Design review of the part shown in the three views and the two pictorial views. Dimensions are in mm from the part's minimum x, y and z. A direction names the side the tool comes from. Give positions to 0.01 mm unless a question says otherwise; leave off trailing zeros. Loops run counter-clockwise (first coordinate to the right, second up) from the corner with the lowest first, then second, coordinate; pieces in that order, holes last. Notation, with made-up numbers: (46.25, 86) -> (99.25, 86) arc R10 cw to (99.25, 91) -> close; hole circle Ø2 at (-25, 40). An arc over 180 degrees is marked (long way). One line per question, with ' | ' between items. Start each with the question number.
(1) Consider section C-C (z = 17.25). Write out the cut boundary in (x, y), and give its area (3 significant figures).
(2) Consider section D-D (z = 12.25). Write out the cut boundary in (x, y) (3 decimals).
(3) Wall thickness on probe 1 along Z at (x, y) = (19.37, 0.85); probe 2 along X at (y, z) = (0.4, 7.25); probe 3 along Z at (x, y) = (14.37, 1.05) (3 decimals): over which ranges is each line inside the solid? List them lowest first.
(4) Consider section A-A (y = 5.75). Write out the cut boundary in (x, z), and give its area (3 significant figures).
(5) Insertion check: P1, Ø8, axis at x = 12, z = 36.5, coming from the +Y side; P2, Ø0.5, axis at x = 1, z = 26, coming from the +Y side. Each pin has a flat end and moves straight along its axis. Give the tip position at first contact, or say it passes through.
(6) Draft analysis for pull direction X (two halves, no side actions). For the marked faces 3, 4, 5 and 6, state which applies: +X half, -X half, draft (parallel to the pull), parting line (faces both ways), or undercut.
(7) Tool access review of the marked faces 1 and 2: name each direction out of +Z, -Z, +X, -X, +Y, -Y from which nothing blocks a thin tool from reaching the whole face with its end or side.
(8) Consider section B-B (x = 14.37). Write out the cut boundary in (y, z) (3 decimals).
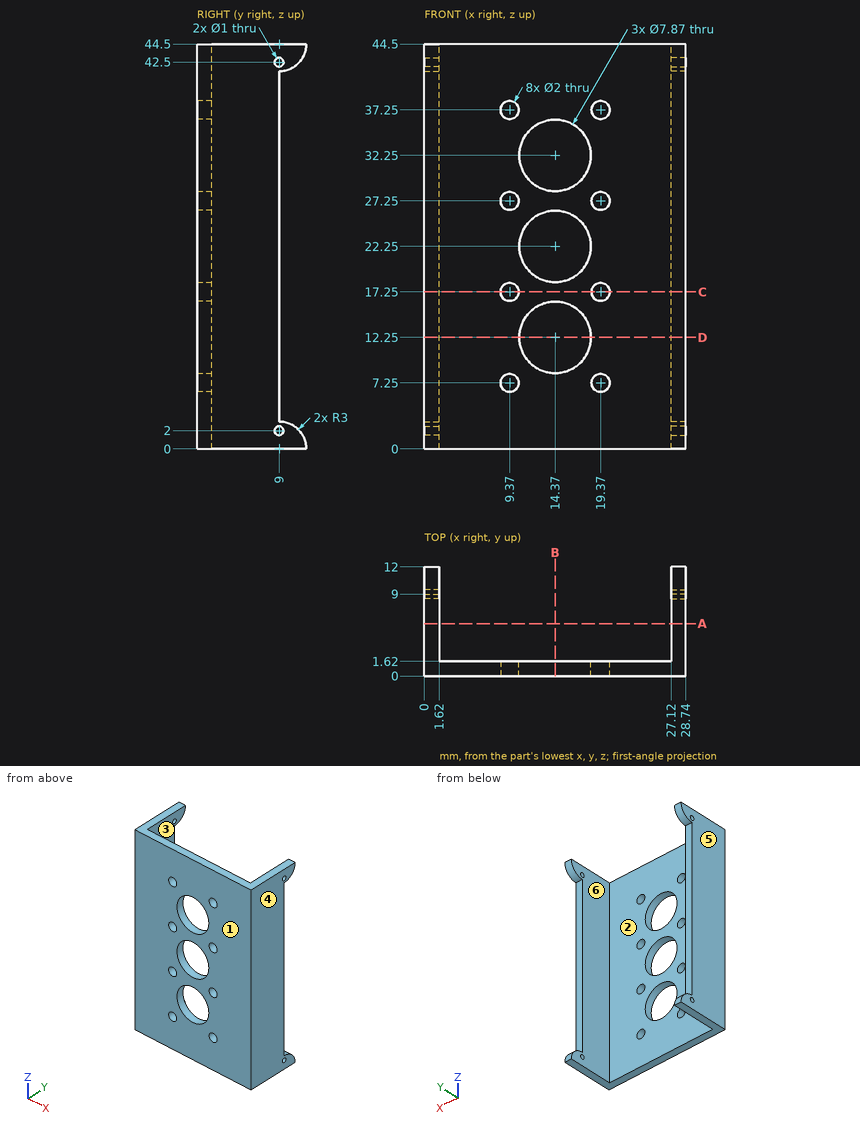
A:
1) outline: (0, 0) -> (8.37, 0) -> (8.37, 1.62) -> (1.62, 1.62) -> (1.62, 9) -> (0, 9) -> close; (10.37, 0) -> (18.37, 0) -> (18.37, 1.62) -> (10.37, 1.62) -> close; (20.37, 0) -> (28.74, 0) -> (28.74, 9) -> (27.12, 9) -> (27.12, 1.62) -> (20.37, 1.62) -> close | area: 64.0 mm^2
2) outline: (0, 0) -> (10.435, 0) -> (10.435, 1.62) -> (1.62, 1.62) -> (1.62, 9) -> (0, 9) -> close; (18.305, 0) -> (28.74, 0) -> (28.74, 9) -> (27.12, 9) -> (27.12, 1.62) -> (18.305, 1.62) -> close
3) probe 1: z = 0 to 6.25, 8.25 to 16.25, 18.25 to 26.25, 28.25 to 36.25, 38.25 to 44.5 | probe 2: x = 0 to 8.37, 10.37 to 18.37, 20.37 to 28.74 | probe 3: z = 0 to 8.315, 16.185 to 18.315, 26.185 to 28.315, 36.185 to 44.5
4) outline: (0, 0) -> (1.62, 0) -> (1.62, 44.5) -> (0, 44.5) -> close; (27.12, 0) -> (28.74, 0) -> (28.74, 44.5) -> (27.12, 44.5) -> close | area: 144 mm^2
5) P1: stops at y = 1.62 | P2: stops at y = 9
6) face 3: undercut | face 4: +X half | face 5: -X half | face 6: undercut
7) face 1: +Z, -Z, +X, -X, -Y | face 2: +Z, -Z, +Y
8) outline: (0, 0) -> (1.62, 0) -> (1.62, 8.315) -> (0, 8.315) -> close; (0, 16.185) -> (1.62, 16.185) -> (1.62, 18.315) -> (0, 18.315) -> close; (0, 26.185) -> (1.62, 26.185) -> (1.62, 28.315) -> (0, 28.315) -> close; (0, 36.185) -> (1.62, 36.185) -> (1.62, 44.5) -> (0, 44.5) -> close
